Design review of the part built by this model. Coordinates are the model's own, in mm. A direction names the side the tool comes from. Coordinates: 2 decimals unless noted, no trailing zeros. Order: outer loops, then holes, each group sorted by start corner. A loop starts at its lowest first (then second) coordinate and runs counter-clockwise, first axis right, second up. Notation, with made-up numbers: (-30, -7) -> (10, -7) arc R12 cw to (10, 6) -> close; hole circle Ø8 at (82, -13). An arc over 180 degrees is marked (long way). Use a Markdown table: item, result. Add a question column.
Q1. Wall thickness on probe 1 along Z at (x, y) = (0.25, 74); probe 2 along Y at (x, z) = (0.25, 10.5); probe 3 along Y at (x, z) = (0.55, 6.25): over which ranges is each line inside the solid? List them lowest first.
Q2. Machinability: for faces 1 (the face through (0, 91.359, 20)), 2 (the face through (0, 80, 21)), 3 (the face through (-1, 12, 0)), which of the approach directions +Z, -Z, +X, -X, +Y, -Y give a long, thin tool a straight path to every point of the face, cutting with its end or side? Answer none if there is none.
Q3. Add section B-B (y = 72). State the section outline as (x, z) points.
Q4. Add section A-A (x = 0). State the section outline as (y, z) points, then the cut area to 3 significant figures.
from build123d import *

# Parameters (mm, degrees)
SWEEP1_PROFILE_R = 1


with BuildPart() as part:
    # Sweep1: sweep along a path in Sketch2
    with BuildLine(Plane(origin=(0, 0, 0), x_dir=(0, 0, -1), z_dir=(1, 0, 0))) as sweep1_path:
        Line((-20, 91.358983849), (-20, 69.358983849))
        ThreePointArc((-20, 69.358983849), (-19.318516526, 64.182602947), (-17.320508076, 59.358983849))
        Line((-17.320508076, 59.358983849), (-2.679491924, 34))
        ThreePointArc((-2.679491924, 34), (-0.681483474, 29.176380902), (0, 24))
        Line((0, 24), (0, 2))
        Line((0, 2), (0, 0))
    # Sweep1 profile (on start of the path) → Sweep1 (sweep)
    with BuildSketch(Plane(origin=(0, 91.358983849, 20), x_dir=(0, 0, -1), z_dir=(0, -1, 0))):
        Circle(SWEEP1_PROFILE_R)
    sweep(path=sweep1_path.line)


solid = part.part
Established:
| question | item | result |
|---|---|---|
| 1 | probe 1 | 19.03 to 20.97 |
| 1 | probe 2 | 45.61 to 49.48 |
| 1 | probe 3 | 38.51 to 41.85 |
| 2 | face 1 | +Z, -Z, +X, -X, +Y |
| 2 | face 2 | +Y |
| 2 | face 3 | -Y |
| 3 | outline | circle Ø2 at (0, 20) |
| 4 | outline | (0, -1) -> (24, -1) arc R21 ccw to (34.5, 1.81) -> (59.86, 16.45) arc R19 cw to (69.36, 19) -> (91.36, 19) -> (91.36, 21) -> (69.36, 21) arc R21 ccw to (58.86, 18.19) -> (33.5, 3.55) arc R19 cw to (24, 1) -> (0, 1) -> close |
| 4 | area | 192 mm^2 |
